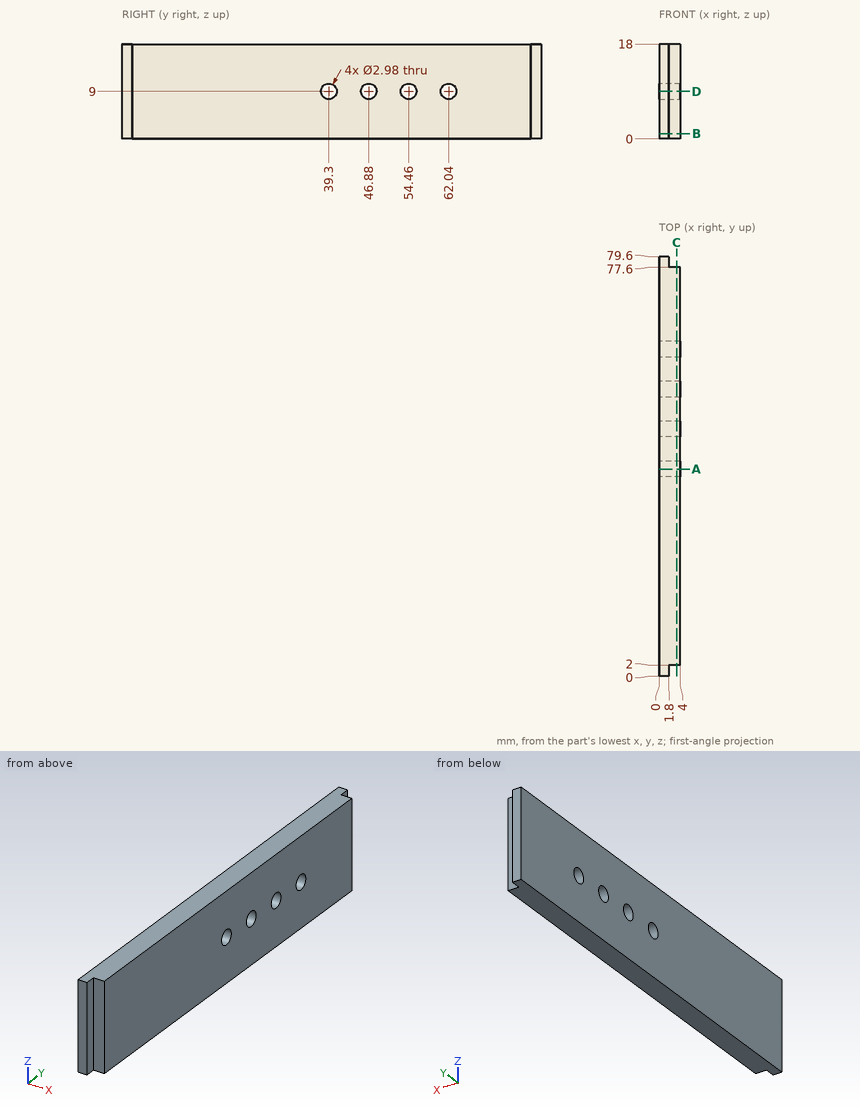
Study the drawing (mm; zero at the part's minimum x, y, z) and answer. Coordinates: 2 decimals unless noted, no trailing zeros. Loops run counter-clockwise (first coordinate to the right, second up) from the corner with the lowest first, then second, coordinate; pieces in that order, holes last. Notation, with made-up numbers: (23.5, 13.5) -> (39.5, 13.5) arc R16 ccw to (39.5, 25.5) -> close; hole circle Ø2 at (-21, 36). An arc over 180 degrees is marked (long way). Write item = value, one per line. Start each with the question number.
1) The part is cut by section B-B, the plane z = 1. Determine the outline of the cut face in (x, y).
2) Find the intervals of material crossed by L1, parallel to Y at x = 1.1, z = 9; L2, parallel to Y at x = 2.05, z = 9; L3, parallel to Z at x = 0.85, y = 46.88, in increasing order. Write a range as from..to.
3) The part is cut by section C-C, the plane x = 3.35. Determine the outline of the cut face in (y, z), plus the area to 3 significant figures.
4) The part is cut by section D-D, the plane z = 9. Determine the outline of the cut face in (x, y).
5) The part is cut by section A-A, the plane y = 39.3. Determine the outline of the cut face in (x, z).
6) Given P1, Ø1.1, axis at x = 3, z = 11, coming from the -Y side; P2, Ø1.6, axis at y = 0.5, z = 12, coming from the +X side; P3, Ø1.8, axis at x = 3.5, z = 12.5, coming from the +Y side, each flat-ended and moving along its own axis, determine where each tip first touches the part or whether it passes through.
Result:
q1.outline = (0, 0) -> (1.8, 0) -> (1.8, 2) -> (4, 2) -> (4, 77.6) -> (1.8, 77.6) -> (1.8, 79.6) -> (0, 79.6) -> close
q2.L1 = 0..37.81, 40.79..45.39, 48.37..52.97, 55.95..60.55, 63.53..79.6
q2.L2 = 2..37.81, 40.79..45.39, 48.37..52.97, 55.95..60.55, 63.53..77.6
q2.L3 = 0..7.51, 10.49..18
q3.outline = (2, 0) -> (77.6, 0) -> (77.6, 18) -> (2, 18) -> close; hole circle Ø2.98 at (39.3, 9); hole circle Ø2.98 at (46.88, 9); hole circle Ø2.98 at (54.46, 9); hole circle Ø2.98 at (62.04, 9)
q3.area = 1,330 mm²
q4.outline = (0, 0) -> (1.8, 0) -> (1.8, 2) -> (4, 2) -> (4, 37.81) -> (0, 37.81) -> close; (0, 40.79) -> (4, 40.79) -> (4, 45.39) -> (0, 45.39) -> close; (0, 48.37) -> (4, 48.37) -> (4, 52.97) -> (0, 52.97) -> close; (0, 55.95) -> (4, 55.95) -> (4, 60.55) -> (0, 60.55) -> close; (0, 63.53) -> (4, 63.53) -> (4, 77.6) -> (1.8, 77.6) -> (1.8, 79.6) -> (0, 79.6) -> close
q5.outline = (0, 0) -> (4, 0) -> (4, 7.51) -> (0, 7.51) -> close; (0, 10.49) -> (4, 10.49) -> (4, 18) -> (0, 18) -> close
q6.P1 = 2
q6.P2 = 1.8
q6.P3 = 77.6
